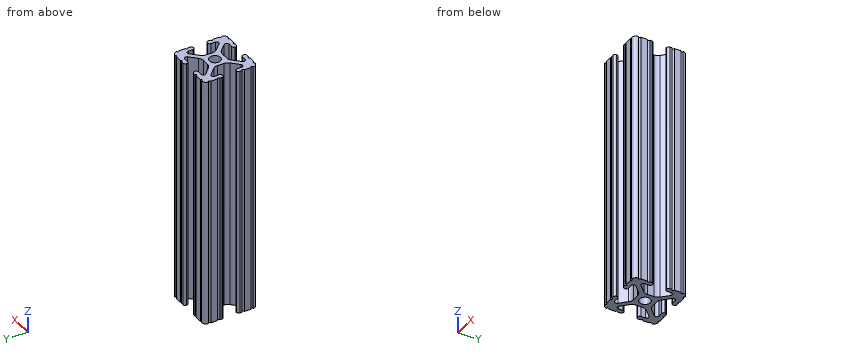
```python
from build123d import *

# Parameters (mm, degrees)
F0_R     = 2.6035
F1_DEPTH = 120


# Not quite as in the source:
# - ends of sketch curves that miss each other by under 0.0002 mm in the source are joined


with BuildPart() as f1:
    # F0 (on Top) → F1 (new body)
    with BuildSketch(Plane.XY):
        with BuildLine():
            ThreePointArc((-3.9522606035, -5.4236922052), (-2.9229262099, -4.7369294977), (-1.7092422, -4.4958))
            Line((-1.7092422, -4.4958), (1.7092422, -4.4958))
            ThreePointArc((1.7092422, -4.4958), (2.9229262099, -4.7369294977), (3.9522606035, -5.4236922052))
            Line((3.9522606035, -5.4236922052), (7.1796402, -8.6451948))
            ThreePointArc((7.1796402, -8.6451948), (7.4147391594, -9.822808991), (6.416421, -10.4902))
            Line((6.416421, -10.4902), (4.28752, -10.4902))
            ThreePointArc((4.28752, -10.4902), (3.5457508444, -10.7974508444), (3.2385, -11.53922))
            Line((3.2385, -11.53922), (3.2385, -11.65098))
            ThreePointArc((3.2385, -11.65098), (3.5457508444, -12.3927491556), (4.28752, -12.7))
            Line((4.28752, -12.7), (5.3171344, -12.7))
            ThreePointArc((5.3171344, -12.7), (5.8251344, -12.192), (6.3331344, -12.7))
            Line((6.3331344, -12.7), (9.5504508, -12.7))
            ThreePointArc((9.5504508, -12.7), (10.0583746, -12.1920000057), (10.5664507771, -12.6998476))
            ThreePointArc((10.5664507771, -12.6998476), (12.0825404752, -12.0825045568), (12.6998469825, -10.5664000074))
            ThreePointArc((12.6998469825, -10.5664000074), (12.1920000057, -10.0583238), (12.7, -9.5504))
            Line((12.7, -9.5504), (12.7, -6.3330836))
            ThreePointArc((12.7, -6.3330836), (12.192, -5.8250836), (12.7, -5.3170836))
            Line((12.7, -5.3170836), (12.7, -4.2874692))
            ThreePointArc((12.7, -4.2874692), (12.3927491556, -3.5457000444), (11.65098, -3.2384492))
            Line((11.65098, -3.2384492), (11.53922, -3.2384492))
            ThreePointArc((11.53922, -3.2384492), (10.7974508444, -3.5457000444), (10.4902, -4.2874692))
            Line((10.4902, -4.2874692), (10.4902, -6.4020954))
            ThreePointArc((10.4902, -6.4020954), (9.8565053438, -7.3510699477), (8.7371366164, -7.1294051977))
            Line((8.7371366164, -7.1294051977), (5.4410102, -3.8408102))
            ThreePointArc((5.4410102, -3.8408102), (4.7508771577, -2.8098852335), (4.5085, -1.5931896))
            Line((4.5085, -1.5931896), (4.5085, 1.5931896))
            ThreePointArc((4.5085, 1.5931896), (4.7508771577, 2.8098852335), (5.4410028439, 3.840817573))
            Line((5.4410028439, 3.840817573), (8.7371428, 7.129399))
            ThreePointArc((8.7371428, 7.129399), (9.8565053438, 7.3510699477), (10.4902, 6.4020954))
            Line((10.4902, 6.4020954), (10.4902, 4.2874692))
            ThreePointArc((10.4902, 4.2874692), (10.7974508444, 3.5457000444), (11.53922, 3.2384492))
            Line((11.53922, 3.2384492), (11.65098, 3.2384492))
            ThreePointArc((11.65098, 3.2384492), (12.3927491556, 3.5457000444), (12.7, 4.2874692))
            Line((12.7, 4.2874692), (12.7, 5.3170836))
            ThreePointArc((12.7, 5.3170836), (12.192, 5.8250836), (12.7, 6.3330836))
            Line((12.7, 6.3330836), (12.7, 9.5504))
            ThreePointArc((12.7, 9.5504), (12.1920000057, 10.0583238), (12.6998476, 10.5663999771))
            ThreePointArc((12.6998476, 10.5663999771), (12.0825404752, 12.0825045568), (10.5664508001, 12.6998475939))
            ThreePointArc((10.5664508001, 12.6998475939), (10.0583746, 12.1920000057), (9.5504508, 12.7))
            Line((9.5504508, 12.7), (6.3331344, 12.7))
            ThreePointArc((6.3331344, 12.7), (5.8251344, 12.192), (5.3171344, 12.7))
            Line((5.3171344, 12.7), (4.28752, 12.7))
            ThreePointArc((4.28752, 12.7), (3.5457508444, 12.3927491556), (3.2385, 11.65098))
            Line((3.2385, 11.65098), (3.2385, 11.53922))
            ThreePointArc((3.2385, 11.53922), (3.5457508444, 10.7974508444), (4.28752, 10.4902))
            Line((4.28752, 10.4902), (6.4767968, 10.4902))
            ThreePointArc((6.4767968, 10.4902), (7.4322289723, 9.8514044384), (7.2070407772, 8.7243726366))
            Line((7.2070407772, 8.7243726366), (3.898265, 5.4231794))
            ThreePointArc((3.898265, 5.4231794), (2.8691189654, 4.7367887684), (1.6557752, 4.4958))
            Line((1.6557752, 4.4958), (-1.6557752, 4.4958))
            ThreePointArc((-1.6557752, 4.4958), (-2.8691189654, 4.7367887684), (-3.8982723561, 5.423172027))
            Line((-3.8982723561, 5.423172027), (-7.2070468, 8.7243666))
            ThreePointArc((-7.2070468, 8.7243666), (-7.4322289723, 9.8514044384), (-6.4767968, 10.4902))
            Line((-6.4767968, 10.4902), (-4.28752, 10.4902))
            ThreePointArc((-4.28752, 10.4902), (-3.5457508444, 10.7974508444), (-3.2385, 11.53922))
            Line((-3.2385, 11.53922), (-3.2385, 11.65098))
            ThreePointArc((-3.2385, 11.65098), (-3.5457508444, 12.3927491556), (-4.28752, 12.7))
            Line((-4.28752, 12.7), (-5.3171344, 12.7))
            ThreePointArc((-5.3171344, 12.7), (-5.8251344, 12.192), (-6.3331344, 12.7))
            Line((-6.3331344, 12.7), (-9.5504508, 12.7))
            ThreePointArc((-9.5504508, 12.7), (-10.0583746, 12.1920000057), (-10.5664507771, 12.6998476))
            ThreePointArc((-10.5664507771, 12.6998476), (-12.0825404752, 12.0825045568), (-12.6998469825, 10.5664000074))
            ThreePointArc((-12.6998469825, 10.5664000074), (-12.1920000057, 10.0583238), (-12.7, 9.5504))
            Line((-12.7, 9.5504), (-12.7, 6.3330836))
            ThreePointArc((-12.7, 6.3330836), (-12.192, 5.8250836), (-12.7, 5.3170836))
            Line((-12.7, 5.3170836), (-12.7, 4.2874692))
            ThreePointArc((-12.7, 4.2874692), (-12.3927491556, 3.5457000444), (-11.65098, 3.2384492))
            Line((-11.65098, 3.2384492), (-11.53922, 3.2384492))
            ThreePointArc((-11.53922, 3.2384492), (-10.7974508444, 3.5457000444), (-10.4902, 4.2874692))
            Line((-10.4902, 4.2874692), (-10.4902, 6.4020954))
            ThreePointArc((-10.4902, 6.4020954), (-9.8565053438, 7.3510699477), (-8.7371366164, 7.1294051977))
            Line((-8.7371366164, 7.1294051977), (-5.4410102, 3.8408102))
            ThreePointArc((-5.4410102, 3.8408102), (-4.7508771577, 2.8098852335), (-4.5085, 1.5931896))
            Line((-4.5085, 1.5931896), (-4.5085, -1.5931896))
            ThreePointArc((-4.5085, -1.5931896), (-4.7508771577, -2.8098852335), (-5.4410028439, -3.840817573))
            Line((-5.4410028439, -3.840817573), (-8.7371428, -7.129399))
            ThreePointArc((-8.7371428, -7.129399), (-9.8565053438, -7.3510699477), (-10.4902, -6.4020954))
            Line((-10.4902, -6.4020954), (-10.4902, -4.2874692))
            ThreePointArc((-10.4902, -4.2874692), (-10.7974508444, -3.5457000444), (-11.53922, -3.2384492))
            Line((-11.53922, -3.2384492), (-11.65098, -3.2384492))
            ThreePointArc((-11.65098, -3.2384492), (-12.3927491556, -3.5457000444), (-12.7, -4.2874692))
            Line((-12.7, -4.2874692), (-12.7, -5.3170836))
            ThreePointArc((-12.7, -5.3170836), (-12.192, -5.8250836), (-12.7, -6.3330836))
            Line((-12.7, -6.3330836), (-12.7, -9.5504))
            ThreePointArc((-12.7, -9.5504), (-12.1920000057, -10.0583238), (-12.6998476, -10.5663999771))
            ThreePointArc((-12.6998476, -10.5663999771), (-12.0825404752, -12.0825045568), (-10.5664508001, -12.6998475939))
            ThreePointArc((-10.5664508001, -12.6998475939), (-10.0583746, -12.1920000057), (-9.5504508, -12.7))
            Line((-9.5504508, -12.7), (-6.3331344, -12.7))
            ThreePointArc((-6.3331344, -12.7), (-5.8251344, -12.192), (-5.3171344, -12.7))
            Line((-5.3171344, -12.7), (-4.28752, -12.7))
            ThreePointArc((-4.28752, -12.7), (-3.5457508444, -12.3927491556), (-3.2385, -11.65098))
            Line((-3.2385, -11.65098), (-3.2385, -11.53922))
            ThreePointArc((-3.2385, -11.53922), (-3.5457508444, -10.7974508444), (-4.28752, -10.4902))
            Line((-4.28752, -10.4902), (-6.416421, -10.4902))
            ThreePointArc((-6.416421, -10.4902), (-7.4147391594, -9.822808991), (-7.1796418951, -8.6451931018))
            Line((-7.1796418951, -8.6451931018), (-3.9522606035, -5.4236922052))
        make_face()
        Circle(F0_R, mode=Mode.SUBTRACT)
    extrude(amount=F1_DEPTH)


solid = f1.part
```
Geometry: final body of the model. Coordinates: model frame, mm. Coordinates: 2 decimals unless noted, no trailing zeros. Order: outer loops, then holes, each group sorted by start corner. A loop starts at its lowest first (then second) coordinate and runs counter-clockwise, first axis right, second up. Notation, with made-up numbers: (59.25, 75.5) - (75.25, 75.5) arc R4 cw to (75.25, 81.5) - close; hole circle Ø9 at (82, 65.5). An arc over 180 degrees is marked (long way). Return JSON: item names as keys, results as strings. Group by question number.
1. Cut plane A-A (y = 0). Output: boundary loops of the cut face in (x, z).
2. Cut plane B-B (x = 0). Output: boundary loops of the cut face in (y, z).
3. Material intervals for line 1 along Y through (x, z) = (0, 57.5); line 2 along Y through (x, z) = (-8.25, 93.5); line 3 along X through (y, z) = (10.25, 78), sorted ascending. Write a range as [from, to].
4. Pin query (flat end, axial travel): pin 1 (4 mm diameter, centred on y = -1.5, z = 14.5, fed in from -X); pin 2 (3.5 mm diameter, centred on y = 0.5, z = 55, fed in from +X); pin 3 (1 mm diameter, centred on x = -3, z = 33.5, fed in from -Y). Return the tip coordinate at first contact, or that it passes through.
Resolved:
{
 "1": {"outline": "(-4.51, 0) - (-2.6, 0) - (-2.6, 120) - (-4.51, 120) - close; (2.6, 0) - (4.51, 0) - (4.51, 120) - (2.6, 120) - close"},
 "2": {"outline": "(-4.5, 0) - (-2.6, 0) - (-2.6, 120) - (-4.5, 120) - close; (2.6, 0) - (4.5, 0) - (4.5, 120) - (2.6, 120) - close"},
 "3": {"line 1": "y = [-4.5, -2.6], [2.6, 4.5]", "line 2": "y = [-12.7, -6.64], [6.64, 12.7]", "line 3": "x = [-12.23, -7.14], [7.14, 12.23]"},
 "4": {"pin 1": "stops at x = -12.34", "pin 2": "stops at x = 4.58", "pin 3": "stops at y = -12.34"}
}
